from build123d import *

# Parameters (mm, degrees)
F0_R     = 6.858
F1_DEPTH = 38.1
F2_DEPTH = 19.05
F3_DEPTH = 12.7


with BuildPart() as f1:
    # F0 (on Top) → F1 (new body)
    with BuildSketch(Plane.XY):
        with BuildLine():
            ThreePointArc((25.4, 17.991581587), (12.2888260632, 23.4224076502), (6.858, 36.533581587))
            Line((6.858, 36.533581587), (-6.858, 36.533581587))
            ThreePointArc((-6.858, 36.533581587), (-12.2888260632, 23.4224076502), (-25.4, 17.991581587))
            Line((-25.4, 17.991581587), (-25.4, -39.666418413))
            Line((-25.4, -39.666418413), (-12.192, -39.666418413))
            ThreePointArc((-12.192, -39.666418413), (0, -27.474418413), (12.192, -39.666418413))
            Line((12.192, -39.666418413), (25.4, -39.666418413))
            Line((25.4, -39.666418413), (25.4, 17.991581587))
        make_face()
        Polygon((-12.192, 10.625581587), (12.192, 10.625581587), (12.192, 0), (12.192, -13.758418413), (-12.192, -13.758418413), (-12.192, 0), align=None, mode=Mode.SUBTRACT)
        Polygon((12.192, 0), (12.192, 10.625581587), (-12.192, 10.625581587), (-12.192, 0), (-12.192, -13.758418413), (12.192, -13.758418413), align=None)
        with Locations((0, -1.566418413)):
            Circle(F0_R, mode=Mode.SUBTRACT)
        with BuildLine():
            Line((25.4, 17.991581587), (25.4, 36.533581587))
            Line((25.4, 36.533581587), (6.858, 36.533581587))
            ThreePointArc((6.858, 36.533581587), (12.2888260632, 23.4224076502), (25.4, 17.991581587))
        make_face()
        with BuildLine():
            ThreePointArc((-25.4, 17.991581587), (-12.2888260632, 23.4224076502), (-6.858, 36.533581587))
            Line((-6.858, 36.533581587), (-25.4, 36.533581587))
            Line((-25.4, 36.533581587), (-25.4, 17.991581587))
        make_face()
        with BuildLine():
            Line((-12.192, -39.666418413), (12.192, -39.666418413))
            ThreePointArc((12.192, -39.666418413), (0, -27.474418413), (-12.192, -39.666418413))
        make_face()
        with Locations((0, -1.566418413)):
            Circle(F0_R)
    extrude(amount=F1_DEPTH)

    # F0 (on Top) → F2 (join)
    with BuildSketch(Plane.XY):
        with BuildLine():
            Line((-12.192, -39.666418413), (12.192, -39.666418413))
            ThreePointArc((12.192, -39.666418413), (0, -27.474418413), (-12.192, -39.666418413))
        make_face()
        Polygon((12.192, 0), (12.192, 10.625581587), (-12.192, 10.625581587), (-12.192, 0), (-12.192, -13.758418413), (12.192, -13.758418413), align=None)
        with Locations((0, -1.566418413)):
            Circle(F0_R, mode=Mode.SUBTRACT)
        with BuildLine():
            Line((25.4, 17.991581587), (25.4, 36.533581587))
            Line((25.4, 36.533581587), (6.858, 36.533581587))
            ThreePointArc((6.858, 36.533581587), (12.2888260632, 23.4224076502), (25.4, 17.991581587))
        make_face()
        with BuildLine():
            ThreePointArc((-25.4, 17.991581587), (-12.2888260632, 23.4224076502), (-6.858, 36.533581587))
            Line((-6.858, 36.533581587), (-25.4, 36.533581587))
            Line((-25.4, 36.533581587), (-25.4, 17.991581587))
        make_face()
    extrude(amount=-F2_DEPTH)

    # F0 (on Top) → F3 (join)
    with BuildSketch(Plane.XY):
        with Locations((0, -1.566418413)):
            Circle(F0_R)
    extrude(amount=-F3_DEPTH)


solid = f1.part
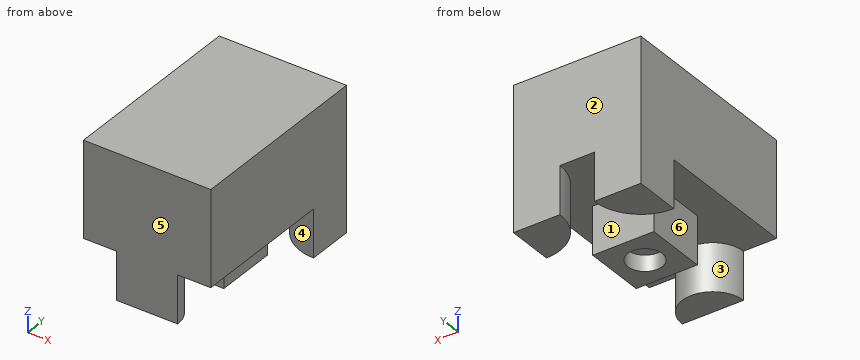
For this review, take the finished solid that the model builds, in its own axes (mm). Face numbers are marked on the shaded views. A direction names the side the tool comes from. Give positions to 0.01 mm unless a question says otherwise; leave off trailing zeros. Order: outer loops, then holes, each group sorted by start corner. A loop starts at its lowest first (then second) coordinate and runs counter-clockwise, first axis right, second up. Notation, with made-up numbers: (15, 7.5) - (50, 7.5) arc R9 cw to (50, 21.5) - close; hole circle Ø7 at (42, 72). An arc over 180 degrees is marked (long way). Answer as a JSON object with one key per item and string values. Group by question number.
Item 1: Clearance check with flat-ended pins moving along their axes: pin 1 Ø5.5 at (x, z) = (0, -5.5) entering from +Y; pin 2 Ø7 at (x, y) = (0, -1) entering from -Z; pin 3 Ø4 at (x, z) = (20, -9.5) entering from -Y. State where each tip first meets the part, or that it passes through.
Item 2: Take a section at D-D on x = -18. Give the boundary of the cut face in (y, z).
Item 3: Wall thickness on line 1 along Y through (x, z) = (0, -15.75); line 2 along Y through (x, z) = (4, -16); line 3 along Z through (x, y) = (18, 3): over which ranges is each line inside the solid? List them lowest first.
Item 4: Take a section at A-A on z = -10. Give the boundary of the cut face in (x, y), and give its area (3 significant figures).
Item 5: Take a section at C-C on y = -33. Give the boundary of the cut face in (x, z), and give its area (3 significant figures).
Item 6: Take a section at B-B on x = 0. Give the boundary of the cut face in (y, z).
Item 7: Draft analysis for pull direction Y (two halves, no side actions). For the marked faces 4, 5 and 6, state which applies: pulls with the +Y half, pulls with the -Y half, needs draft (parallel to the pull), parting line crosses it, or undercut.
Item 8: Machinability: for the marked faces 1, 2 and 3, which of the approach directions +Z, -Z, +X, -X, +Y, -Y give a long, thin tool a straight path to every point of the face, cutting with its end or side? Answer none if there is none.
Reported:
{
 "1": {"pin 1": "y = 10.63", "pin 2": "z = -12.7", "pin 3": "y = 18.31"},
 "2": {"outline": "(-39.67, 0) - (19.53, 0) - (19.53, -19.05) - (36.53, -19.05) - (36.53, 38.1) - (-39.67, 38.1) - close"},
 "3": {"line 1": "-39.67 to -27.47, -13.76 to -8.42, 5.29 to 10.63", "line 2": "-39.67 to -28.15, -13.76 to -7.14, 4 to 10.63", "line 3": "0 to 38.1"},
 "4": {"outline": "(-25.4, 17.99) arc R18.54 ccw to (-6.86, 36.53) - (-25.4, 36.53) - close; (-12.19, -39.67) - (12.19, -39.67) arc R12.19 ccw to start; (-12.19, -13.76) - (12.19, -13.76) - (12.19, 10.63) - (-12.19, 10.63) - close; (6.86, 36.53) arc R18.54 ccw to (25.4, 17.99) - (25.4, 36.53) - close", "area": "1,370 mm^2"},
 "5": {"outline": "(-25.4, 0) - (-10.21, 0) - (-10.21, -19.05) - (10.21, -19.05) - (10.21, 0) - (25.4, 0) - (25.4, 38.1) - (-25.4, 38.1) - close", "area": "2,320 mm^2"},
 "6": {"outline": "(-39.67, -19.05) - (-27.47, -19.05) - (-27.47, 0) - (-13.76, 0) - (-13.76, -19.05) - (-8.42, -19.05) - (-8.42, -12.7) - (5.29, -12.7) - (5.29, -19.05) - (10.63, -19.05) - (10.63, 0) - (36.53, 0) - (36.53, 38.1) - (-39.67, 38.1) - close"},
 "7": {"face 4": "undercut", "face 5": "pulls with the -Y half", "face 6": "needs draft"},
 "8": {"face 1": "-Z, +X, -X", "face 2": "+Z, -Z, +X, -X, +Y", "face 3": "-Z"}
}
